from build123d import *

# Parameters (mm, degrees)
F0_W     = 50.8
F0_H     = 76.2
F1_DEPTH = 33.782
F2_R     = 6.35
F3_DEPTH = 16.002
F4_T     = -2.54


with BuildPart() as f1:
    # F0 (on Top) → F1 (new body)
    with BuildSketch(Plane.XY):
        with Locations((25.4, 38.1)):
            Rectangle(F0_W, F0_H)
    extrude(amount=F1_DEPTH)

    # F2 (on face) → F3 (cut)
    with BuildSketch(Plane.XY.offset(33.782)):
        with Locations((25.4, 38.1)):
            Circle(F2_R)
    extrude(amount=-F3_DEPTH, mode=Mode.SUBTRACT)

    # F4
    f4_openings = [f1.faces().sort_by_distance(p)[0] for p in [
        (0, 38.1, 16.891),
    ]]
    offset(amount=F4_T, openings=f4_openings, kind=Kind.INTERSECTION)


solid = f1.part
Can you work these out from the model? Positions are in its coordinate system, mm. A direction names the side the tool comes from. Give positions to 0.01 mm unless a question says otherwise; leave off trailing zeros. Write each loop counter-clockwise with the first axis right and the second up, starting at its lowest first coordinate (ties: lowest second). Pieces come first, ordered by that corner, then holes. Notation, with made-up numbers: (-13.75, 85.25) -> (25.25, 85.25) arc R30 ccw to (25.25, 109.25) -> close; hole circle Ø3 at (-29.5, 16). An arc over 180 degrees is marked (long way). Answer as a JSON object with one key per item and string values. Group by question number.
Item 1: Suppose I cut it at B-B (z = 29.5). Please give me the cut outline in (x, y).
Item 2: I'm going to push flat-ended pins straight in: P1, Ø7.5, axis at x = 25.4, y = 38.1, coming from the +Z side; P2, Ø1, axis at y = 46, z = 8, coming from the -X side; P3, Ø1.5, axis at y = 30, z = 20.5, coming from the -X side. Where does each tip first touch, or does it pass through?
Item 3: Suppose I cut it at A-A (z = 16.5). Please give me the cut outline in (x, y).
Item 4: Suppose I cut it at C-C (x = 25.4). Please give me the cut outline in (y, z), plus the area to 3 significant figures.
Item 5: For faces 1 (the face through (18, 47, 31.242)), 2 (the face through (25, 38, 15.24)), 3 (the face through (25, 38, 17.78)), 4 (the face through (25, 47, 33.782)), which set-ups out of +Z, -Z, +X, -X, +Y, -Y let a thin tool reach every point of the face, with its end or its side?
Item 6: Suppose I cut it at D-D (y = 6). Please give me the cut outline in (x, z).
Item 7: We'd pull the mould along Y, two halves only. Please class faces 5 (the face through (25, 39, 0)), 6 (the face through (25, 0, 17)), 7 (the face through (24, 2.54, 17)): +Y half, -Y half, draft (parallel to the pull), parting line (faces both ways), or undercut.
Item 8: Please list where these lines run through material, in increasing order: line 1 (X direction, y = 38, z = 28); line 2 (Y direction, x = 25, z = 28); line 3 (Y direction, x = 42, z = 25). Write a range as [from, to].
Findings:
{
 "1": {"outline": "(0, 0) -> (50.8, 0) -> (50.8, 76.2) -> (0, 76.2) -> (0, 73.66) -> (48.26, 73.66) -> (48.26, 2.54) -> (0, 2.54) -> close; circle Ø17.78 at (25.4, 38.1); hole circle Ø12.7 at (25.4, 38.1)"},
 "2": {"P1": "stops at z = 17.78", "P2": "stops at x = 48.26", "P3": "stops at x = 20.4"},
 "3": {"outline": "(0, 0) -> (50.8, 0) -> (50.8, 76.2) -> (0, 76.2) -> (0, 73.66) -> (48.26, 73.66) -> (48.26, 2.54) -> (0, 2.54) -> close; circle Ø17.78 at (25.4, 38.1)"},
 "4": {"outline": "(0, 0) -> (76.2, 0) -> (76.2, 33.78) -> (44.45, 33.78) -> (44.45, 17.78) -> (31.75, 17.78) -> (31.75, 33.78) -> (0, 33.78) -> close; hole (2.54, 2.54) -> (73.66, 2.54) -> (73.66, 31.24) -> (46.99, 31.24) -> (46.99, 15.24) -> (29.21, 15.24) -> (29.21, 31.24) -> (2.54, 31.24) -> close", "area": "614 mm²"},
 "5": {"face 1": "none", "face 2": "-X", "face 3": "+Z", "face 4": "+Z, +X, -X, +Y, -Y"},
 "6": {"outline": "(0, 0) -> (50.8, 0) -> (50.8, 33.78) -> (0, 33.78) -> (0, 31.24) -> (48.26, 31.24) -> (48.26, 2.54) -> (0, 2.54) -> close"},
 "7": {"face 5": "draft", "face 6": "-Y half", "face 7": "undercut"},
 "8": {"line 1": "x = [16.51, 19.05], [31.75, 34.29], [48.26, 50.8]", "line 2": "y = [0, 2.54], [29.22, 31.76], [44.44, 46.98], [73.66, 76.2]", "line 3": "y = [0, 2.54], [73.66, 76.2]"}
}
